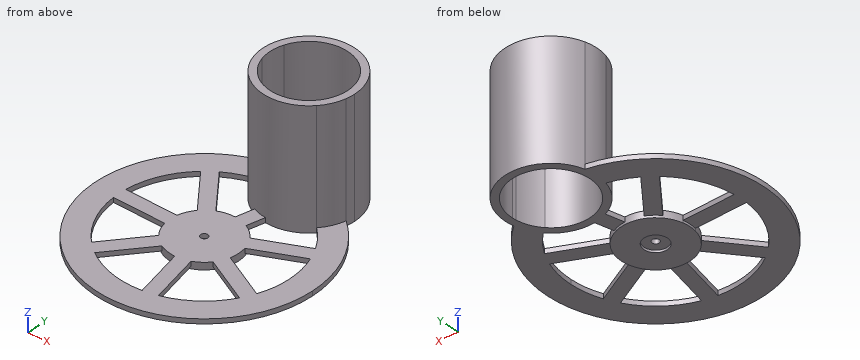
from build123d import *

# Parameters (mm, degrees)
F1_DEPTH = 2
F0_R     = 5
F0_R_2   = 1.5
F2_DEPTH = 2
F3_COUNT = 7
F4_DEPTH = 25
F5_DEPTH = 50
F6_DEPTH = 1


with BuildPart() as f1:
    # F0 (on Top) → F1 (new body)
    with BuildSketch(Plane.XY):
        with BuildLine():
            ThreePointArc((-9.6980178026, 35.1732821843), (-10.4180475342, 40.3053577212), (-9.7713618559, 45.4471900565))
            ThreePointArc((-9.7713618559, 45.4471900565), (-29.212132235, -36.1604469944), (46.4857676773, 0))
            ThreePointArc((46.4857676773, 0), (41.7541400396, 20.4332666527), (28.5224895833, 36.7068683562))
            ThreePointArc((28.5224895833, 36.7068683562), (26.8741758072, 31.793651098), (23.9987273116, 27.4822200037))
            ThreePointArc((23.9987273116, 27.4822200037), (33.217640994, 15.0930333501), (36.4857688546, 0))
            ThreePointArc((36.4857688546, 0), (1.5012714069, -36.4548695386), (-36.3622239269, -3))
            ThreePointArc((-36.3622239269, -3), (-36.4857688546, 0), (-36.3622239269, 3))
            ThreePointArc((-36.3622239269, 3), (-28.0921072309, 23.2818564603), (-9.6980178026, 35.1732821843))
        make_face()
    extrude(amount=F1_DEPTH)



with BuildPart() as f1b:
    # F0 (on Top) → F1, piece 2 (new body)
    with BuildSketch(Plane.XY):
        with BuildLine():
            ThreePointArc((14.7, 0), (1.5079551369, 14.6224509336), (-14.3906219463, 3))
            ThreePointArc((-14.3906219463, 3), (-14.7, 0), (-14.3906219463, -3))
            ThreePointArc((-14.3906219463, -3), (1.5079551369, -14.6224509336), (14.7, 0))
        make_face()
        Circle(F0_R, mode=Mode.SUBTRACT)
        Circle(F0_R)
        Circle(F0_R_2, mode=Mode.SUBTRACT)
    extrude(amount=F1_DEPTH)


with BuildPart() as f2:
    # F0 (on Top) → F2 (new body)
    with BuildSketch(Plane.XY):
        with BuildLine():
            Line((-14.3906219463, 3), (-36.3622239269, 3))
            ThreePointArc((-36.3622239269, 3), (-36.4857688546, 0), (-36.3622239269, -3))
            Line((-36.3622239269, -3), (-14.3906219463, -3))
            ThreePointArc((-14.3906219463, -3), (-14.7, 0), (-14.3906219463, 3))
        make_face()
    extrude(amount=F2_DEPTH)


with BuildPart() as f1_1:
    add(f1.part)

    add(f1b.part)  # F3 merges F1b
    # F3: F2 ×7 about axis
    f3_axis = Axis((0, 0, 2), (0, 0, -1))
    for i in range(1, F3_COUNT):
        add(f2.part.rotate(f3_axis, i * 360 / F3_COUNT))

    # F0 (on Top) → F4 (cut)
    with BuildSketch(Plane.XY):
        with BuildLine():
            ThreePointArc((21.6570841341, 29.3629364288), (8.1188473616, 35.5709944538), (-6.7722579251, 35.851748235))
            ThreePointArc((-6.7722579251, 35.851748235), (5.5264782191, 24.2130831291), (21.6570841341, 29.3629364288))
        make_face()
    extrude(amount=F4_DEPTH, mode=Mode.SUBTRACT)

    # F0 (on Top) → F5 (join)
    with BuildSketch(Plane.XY):
        with BuildLine():
            ThreePointArc((-6.4520489204, 46.03583019), (12.0680177843, 56.8522288954), (25.8814517695, 40.4456328669))
            ThreePointArc((25.8814517695, 40.4456328669), (25.8578955004, 39.5602691783), (25.7872933477, 38.6774106986))
            ThreePointArc((25.7872933477, 38.6774106986), (27.1727600693, 37.7169419064), (28.5224895833, 36.7068683562))
            ThreePointArc((28.5224895833, 36.7068683562), (28.7915053614, 38.5676543049), (28.8814517695, 40.4456328669))
            ThreePointArc((28.8814517695, 40.4456328669), (11.7530794444, 59.9331646211), (-9.7713618559, 45.4471900565))
            ThreePointArc((-9.7713618559, 45.4471900565), (-8.117043095, 45.7716091911), (-6.4520489204, 46.03583019))
        make_face()
        with BuildLine():
            ThreePointArc((-6.7722579251, 35.851748235), (-7.4103241816, 40.9688853837), (-6.4520489204, 46.03583019))
            ThreePointArc((-6.4520489204, 46.03583019), (-8.117043095, 45.7716091911), (-9.7713618559, 45.4471900565))
            ThreePointArc((-9.7713618559, 45.4471900565), (-10.4180475342, 40.3053577212), (-9.6980178026, 35.1732821843))
            ThreePointArc((-9.6980178026, 35.1732821843), (-8.2421219769, 35.5426329108), (-6.7722579251, 35.851748235))
        make_face()
        with BuildLine():
            ThreePointArc((28.5224895833, 36.7068683562), (27.1727600693, 37.7169419064), (25.7872933477, 38.6774106986))
            ThreePointArc((25.7872933477, 38.6774106986), (24.4522045664, 33.6964711194), (21.6570841341, 29.3629364288))
            ThreePointArc((21.6570841341, 29.3629364288), (22.8472657721, 28.4466830343), (23.9987273116, 27.4822200037))
            ThreePointArc((23.9987273116, 27.4822200037), (26.8741758072, 31.793651098), (28.5224895833, 36.7068683562))
        make_face()
        with BuildLine():
            ThreePointArc((21.6570841341, 29.3629364288), (5.5264782191, 24.2130831291), (-6.7722579251, 35.851748235))
            ThreePointArc((-6.7722579251, 35.851748235), (-8.2421219769, 35.5426329108), (-9.6980178026, 35.1732821843))
            ThreePointArc((-9.6980178026, 35.1732821843), (4.8589154172, 21.2882993925), (23.9987273116, 27.4822200037))
            ThreePointArc((23.9987273116, 27.4822200037), (22.8472657721, 28.4466830343), (21.6570841341, 29.3629364288))
        make_face()
    extrude(amount=F5_DEPTH)


    add(f2.part)  # F6 merges F2
    # F0 (on Top) → F6 (join)
    with BuildSketch(Plane.XY):
        with BuildLine():
            ThreePointArc((14.7, 0), (1.5079551369, 14.6224509336), (-14.3906219463, 3))
            ThreePointArc((-14.3906219463, 3), (-14.7, 0), (-14.3906219463, -3))
            ThreePointArc((-14.3906219463, -3), (1.5079551369, -14.6224509336), (14.7, 0))
        make_face()
        Circle(F0_R, mode=Mode.SUBTRACT)
    extrude(amount=-F6_DEPTH)


solid = f1_1.part
Work out the finished part from the listing and answer in its coordinate system (mm). Give positions to 0.01 mm unless a question says otherwise; leave off trailing zeros. Loops run counter-clockwise (first coordinate to the right, second up) from the corner with the lowest first, then second, coordinate; pieces in that order, holes last. Notation, with made-up numbers: M -6.75,-14 L 19.25,-14 A24 cw 19.25,-4 Z; hole C 14,-40 d4. An arc over 180 degrees is marked long. Use CSV: the item, a comma, the result in double quotes.
1) Find section D-D on y = -39.5. Write down the section's boundary in (x, z), plus the area to 3 significant figures.
Answer:
outline,"M -24.51,0 L 24.51,0 L 24.51,2 L -24.51,2 Z"
area,"98.0 mm^2"
2) Find section B-B on z = 46. Write down the section's boundary in (x, y).
Answer:
outline,"C 9.23,40.45 d39.3; hole C 9.23,40.45 d33.3"
3) Consider L1, parallel to Z at x = 12, y = 23.5; L2, parallel to X at y = 27, z = 24; L3, parallel to Z at x = 40.5, y = 12. Determine where each line is inside the solid, lowest interval first.
Answer:
L1,"0 to 50"
L2,"-5.1 to -0.59, 19.05 to 23.56"
L3,"0 to 2"
4) Find section A-A on x = -28. Write down the section's boundary in (y, z).
Answer:
outline,"M -37.11,0 L -23.39,0 L -23.39,2 L -37.11,2 Z; M -3,0 L 3,0 L 3,2 L -3,2 Z; M 23.39,0 L 37.11,0 L 37.11,2 L 23.39,2 Z"
5) Given P1, Ø12, axis at x = -8.5, z = 29, coming from the -Y side; P2, Ø12, axis at x = 31, y = 1.5, coming from the -Z side; P3, Ø12, axis at x = -2, z = 31, coming from the -Y side, each flat-ended and moving along its own axis, determine where each tip first touches the part or whether it passes through.
Answer:
P1,"y = 24.68"
P2,"z = 0"
P3,"y = 21.5"
6) Find section C-C on x = 20. Write down the section's boundary in (y, z), plus the area to 3 significant figures.
Answer:
outline,"M -41.96,0 L -30.52,0 L -30.52,2 L -41.96,2 Z; M -12.96,0 L -6.3,0 L -6.3,2 L -12.96,2 Z; M 6.3,0 L 12.96,0 L 12.96,2 L 6.3,2 Z; M 24.01,0 L 27.75,0 L 27.75,50 L 24.01,50 Z; M 53.14,0 L 56.88,0 L 56.88,50 L 53.14,50 Z"
area,"423 mm^2"
